from build123d import *

# Parameters (mm, degrees)
CHANFREIN2_SIZE         = 0.5
EMPREINTE_POUR_CL_DEPTH = 2.8


with BuildPart() as part:
    # Esquisse1 → Base-Révolution (revolve)
    with BuildSketch(Plane.XY, mode=Mode.PRIVATE) as base_r_volution_sk:
        Polygon((0, 0), (0, 3), (16, 3), (18.5, 5.5), (19, 5.5), (19, 0), align=None)
    revolve(base_r_volution_sk.sketch.rotate(Axis((-25.828475034, 0, 0), (1, 0, 0)), 90), axis=Axis((-25.828475034, 0, 0), (1, 0, 0)))

    # Chanfrein2
    chanfrein2_edges = [part.edges().sort_by_distance(p)[0] for p in [
        (0, 0, -3),
    ]]
    chamfer(chanfrein2_edges, length=CHANFREIN2_SIZE)

    # Esquisse2 → Empreinte pour clé (cut)
    with BuildSketch(Plane(origin=(19, 0, 0), x_dir=(0, 0, -1), z_dir=(1, 0, 0))):
        Polygon((2.309401077, 0), (1.154700538, 2), (-1.154700538, 2), (-2.309401077, 0), (-1.154700538, -2), (1.154700538, -2), align=None)
    extrude(amount=-EMPREINTE_POUR_CL_DEPTH, mode=Mode.SUBTRACT)


solid = part.part
Can you work these out from the model? Positions are in its coordinate system, mm. A direction names the side the tool comes from. Coordinates: 2 decimals unless noted, no trailing zeros. Order: outer loops, then holes, each group sorted by start corner. A loop starts at its lowest first (then second) coordinate and runs counter-clockwise, first axis right, second up. Notation, with made-up numbers: M -19,-39.75 L -15,-39.75 A18 ccw -15,-6.75 Z; hole C 78.25,24 d4. An arc over 180 degrees is marked long. Write item = value, one per line.
(1) Suppose I cut it at C-C on x = 2. Please give me the cut outline in (y, z), plus the area to 3 significant figures.
Results are:
outline = C 0,0 d6
area = 28.3 mm2
(2) Suppose I cut it at B-B on z = 0. Please give me the cut outline in (x, y).
Results are:
outline = M 0,-2.5 L 0.5,-3 L 16,-3 L 18.5,-5.5 L 19,-5.5 L 19,-2 L 16.2,-2 L 16.2,2 L 19,2 L 19,5.5 L 18.5,5.5 L 16,3 L 0.5,3 L 0,2.5 Z
(3) For faces 1 (the face through (19, 2.4, -0.1)), 2 (the face through (16.2, 0, 0)), which set-ups out of +Z, -Z, +X, -X, +Y, -Y let a thin tool reach every point of the face, with its end or its side?
Results are:
face_1 = +Z, -Z, +X, +Y, -Y
face_2 = +X
(4) I need wall thicknesses on line 1 along X through (y, z) = (-0.5, -1.25); line 2 along Z through (x, y) = (16.75, 0.25); line 3 along Y through (x, z) = (18, -4). Which ranges of each line are inside material? Lowest first, please. Write a range as [from, to].
Results are:
line_1 = [0, 16.2]
line_2 = [-3.74, -2.17], [2.17, 3.74]
line_3 = [-3, 3]
(5) If we mould it in two halves opening along Z, with no side actions, what happens to faces 3 (the face through (8.36, -0.9, 2.86)), 4 (the face through (0, 0, 0)), 5 (the face through (17.62, 1.014, 1.724))? For each: pulls with the +Z half, pulls with the -Z half, needs draft (parallel to the pull), parting line crosses it, or undercut.
Results are:
face_3 = parting line crosses it
face_4 = needs draft
face_5 = undercut
(6) Suppose I cut it at A-A on x = 17.5. Please give me the cut outline in (y, z).
Results are:
outline = C 0,0 d9; hole M -2,-1.15 L 0,-2.31 L 2,-1.15 L 2,1.15 L 0,2.31 L -2,1.15 Z
(7) For pin 1 Ø1 at (x, y) = (7, 1.5) entering from -Z; pin 2 Ø1 at (y, z) = (-3, -2.5) entering from -X; pin 3 Ø0.7 at (x, z) = (17.5, -0.5) entering from +Y, each with a flat end and sliding along its axis, tell me the tip position at first contact or that it passes through.
Results are:
pin_1 = -2.83
pin_2 = 16.41
pin_3 = 4.83
